Input: part model. Units: mm. Frame: model coordinates. Face numbers are marked on the shaded views. A direction names the side the tool comes from. Round coordinates to 2 decimals unless told otherwise and drop trailing zeros. Order: outer loops, then holes, each group sorted by start corner. A loop starts at its lowest first (then second) coordinate and runs counter-clockwise, first axis right, second up.
Item 1: First-contact query: pin 1 (1.5 mm diameter, centred on x = 0.5, z = 8, fed in from +Y); pin 2 (1 mm diameter, centred on y = -1.5, z = 9.5, fed in from -X); pin 3 (6 mm diameter, centred on x = -3, z = 12.5, fed in from -Y); pin 4 (4.5 mm diameter, centred on x = 0, y = 0, fed in from +Z). Flat tips, straight axial feed; report the tip coordinate or a pass-through.
Item 2: Reachability of the marked faces 1 and 2 from +Z, -Z, +X, -X, +Y, -Y: full face, straight path, thin tool, end or side. Return the list, or none.
Item 3: Mould query, pull axis Y, two halves, no side actions, for the marked faces 3, 4 and 5. Classes: released by +Y, released by -Y, zero draft, split by the parting line, or undercut.
Item 4: Cut plane C-C on z = 11.5. Output: boundary loops of the cut face in (x, y), then the cut area to 3 significant figures.
Item 5: Cut plane D-D on y = 6.25. Output: boundary loops of the cut face in (x, z), then the cut area to 3 significant figures.
Item 6: Line query: L1, parallel to Y at x = 0, z = 11; L2, parallel to X at y = 1.5, z = 1.25; L3, parallel to Y at x = -3, z = 14.75. Output: solid intervals per line, ascending.
Item 7: Cut plane A-A on x = 0. Output: boundary loops of the cut face in (y, z).
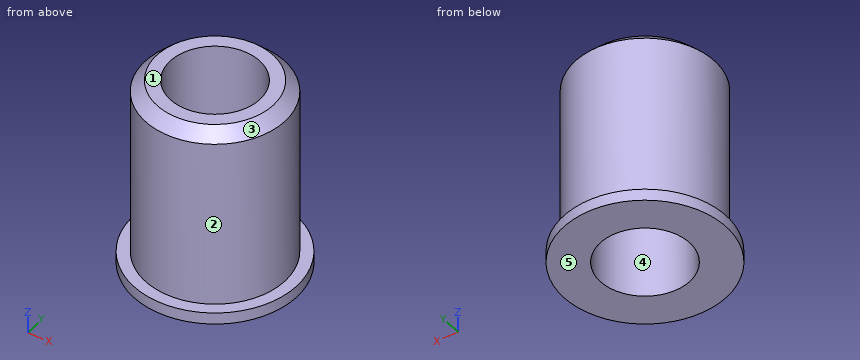
```python
from build123d import *

# Parameters (mm, degrees)
SKETCH_R     = 7
PAD_DEPTH    = 1
SKETCH001_R  = 6
PAD001_DEPTH = 15.5
CHAMFER_SIZE = 1
SKETCH002_R  = 3.85
POCKET_DEPTH = 16.501


with BuildPart() as part:
    # Sketch → Pad (new body)
    with BuildSketch(Plane.XY):
        Circle(SKETCH_R)
    extrude(amount=PAD_DEPTH)

    # Sketch001 (on Face3 of Pad) → Pad001 (join)
    with BuildSketch(Plane.XY.offset(1)):
        Circle(SKETCH001_R)
    extrude(amount=PAD001_DEPTH)

    # Chamfer
    chamfer_edges = [part.edges().sort_by_distance(p)[0] for p in [
        (-6, 0, 16.5),
    ]]
    chamfer(chamfer_edges, length=CHAMFER_SIZE)

    # Sketch002 (on Face4 of Chamfer) → Pocket (cut, through all)
    with BuildSketch(Plane.XY.offset(16.5)):
        Circle(SKETCH002_R)
    extrude(amount=-POCKET_DEPTH, mode=Mode.SUBTRACT)


solid = part.part
```
From the geometry:
1. pin 1: stops at y = 6
1. pin 2: stops at x = -5.92
1. pin 3: stops at y = -6
1. pin 4: passes through
2. face 1: +Z, +X, -X, +Y, -Y
2. face 2: +Z
3. face 3: split by the parting line
3. face 4: undercut
3. face 5: zero draft
4. outline: circle Ø12 at (0, 0); hole circle Ø7.7 at (0, 0)
4. area: 66.5 mm2
5. outline: (-3.15, 0) - (3.15, 0) - (3.15, 1) - (-3.15, 1) - close
5. area: 6.30 mm2
6. L1: y = -6 to -3.85, 3.85 to 6
6. L2: x = -5.81 to -3.55, 3.55 to 5.81
6. L3: y = -5.2 to -2.41, 2.41 to 5.2
7. outline: (-7, 0) - (-3.85, 0) - (-3.85, 16.5) - (-5, 16.5) - (-6, 15.5) - (-6, 1) - (-7, 1) - close; (3.85, 0) - (7, 0) - (7, 1) - (6, 1) - (6, 15.5) - (5, 16.5) - (3.85, 16.5) - close
